```python
from build123d import *

# Parameters (mm, degrees)
SKETCH1_W               = 96.0628
SKETCH1_H               = 90.3478
PCB_DEPTH               = 1.6256
SKETCH5_R               = 1.5875
PCB_HOLES_DEPTH         = 66.957101229
SKETCH2_W               = 7.9756
SKETCH2_H               = 60.2234
PCI_104_CONNECTOR_DEPTH = 9.2964
SKETCH6_W               = 63.5
SKETCH6_H               = 7.366
PCB_EDGE_CONNS_DEPTH    = 5.461


with BuildPart() as part:
    # Sketch1 → PCB (new body)
    with BuildSketch(Plane.XY):
        Rectangle(SKETCH1_W, SKETCH1_H)
    extrude(amount=PCB_DEPTH)

    # Sketch5 → PCB_Holes (cut, through all)
    with BuildSketch(Plane.XY.offset(1.6256)):
        with Locations((-42.7736, 36.83)):
            Circle(SKETCH5_R)
        with Locations((42.9514, 40.005)):
            Circle(SKETCH5_R)
        with Locations((42.9514, -40.005)):
            Circle(SKETCH5_R)
        with Locations((-42.7736, -36.83)):
            Circle(SKETCH5_R)
    extrude(amount=-PCB_HOLES_DEPTH, mode=Mode.SUBTRACT)

    # Sketch2 → PCI-104_Connector (add)
    with BuildSketch(Plane.XY.offset(1.6256)):
        with Locations((-39.6494, 0.4064)):
            Rectangle(SKETCH2_W, SKETCH2_H)
    extrude(amount=PCI_104_CONNECTOR_DEPTH)

    # Sketch6 → PCB_Edge_Conns (add)
    with BuildSketch(Plane.XY.offset(1.6256)):
        with Locations((-3.5814, -46.0629)):
            Rectangle(SKETCH6_W, SKETCH6_H)
    extrude(amount=PCB_EDGE_CONNS_DEPTH)


solid = part.part
```
Source: CAD feature listing. Evaluate the final solid. Frame: model axes, mm. A direction names the side the tool comes from. Round coordinates to 2 decimals unless told otherwise and drop trailing zeros. Write each loop counter-clockwise with the first axis right and the second up, starting at its lowest first coordinate (ties: lowest second). Pieces come first, ordered by that corner, then holes. Notation, with made-up numbers: M 42.25,53.25 L 74.25,53.25 A19 cw 74.25,69.25 Z; hole C 62,-40 d8. An arc over 180 degrees is marked long. Use CSV: the item, a comma, the result in double quotes. Start each with the question number.
Q1. Cut plane B-B on z = 5.25. Output: boundary loops of the cut face in (x, y), plus the area to 3 significant figures.
Q2. Cut plane A-A on y = -36.83. Output: boundary loops of the cut face in (x, z), plus the area to 3 significant figures.
Q3. First-contact query: P1, Ø5, axis at x = 42.95, y = -40.01, coming from the +Z side; P2, Ø1.6, axis at x = 0, z = 5, coming from the +Y side; P3, Ø2.5, axis at x = -39.5, z = 8, coming from the +Y side; P4, Ø3, axis at x = 42.95, y = 40.01, coming from the +Z side. Flat tips, straight axial feed; report the tip coordinate or a pass-through.
Q4. Pull-direction query (Y, two-part tool) for faces 5 (the face through (-40, 1, 10.922)), 6 (the face through (43.684, 38.597, 0.824)), 7 (the face through (-4, -42.38, 4)); classes: +Y half, -Y half, draft (parallel to the pull), parting line (faces both ways), or undercut.
Q5. Line query: line 1 (Y direction, x = -30, z = 5.5); line 2 (X direction, y = -12.5, z = 2.75); line 3 (Z direction, x = 23.5, y = 27). Output: solid intervals per line, ascending. Write a range as from..to.
Q6. Cut plane C-C on x = -27.5. Output: boundary loops of the cut face in (y, z), plus the area to 3 significant figures.
Q7. Access query for faces 1 (the face through (-40, 30.518, 6)), 2 (the face through (-43.637, 0, 6)), 3 (the face through (-40, -29.705, 6)), 4 (the face through (28.169, -46, 4)). Directions: +Z, -Z, +X, -X, +Y, -Y. A direction counts if a zero-diameter tool reaches every point of the face in a straight line with its end or side. Return the directions, or none.
Q8. Cut plane D-D on y = 5.5. Output: boundary loops of the cut face in (x, z), plus the area to 3 significant figures.
Results found:
1,outline,"M -43.64,-29.71 L -35.66,-29.71 L -35.66,30.52 L -43.64,30.52 Z; M -35.33,-49.75 L 28.17,-49.75 L 28.17,-42.38 L -35.33,-42.38 Z"
1,area,"948 mm^2"
2,outline,"M -48.03,0 L -44.36,0 L -44.36,1.63 L -48.03,1.63 Z; M -41.19,0 L 48.03,0 L 48.03,1.63 L -41.19,1.63 Z"
2,area,"151 mm^2"
3,P1,"z = 1.63"
3,P2,"y = -42.38"
3,P3,"y = 30.52"
3,P4,"through"
4,face 5,"draft"
4,face 6,"undercut"
4,face 7,"+Y half"
5,line 1,"-49.75..-42.38"
5,line 2,"-43.64..-35.66"
5,line 3,"0..1.63"
6,outline,"M -49.75,1.63 L -45.17,1.63 L -45.17,0 L 45.17,0 L 45.17,1.63 L -42.38,1.63 L -42.38,7.09 L -49.75,7.09 Z"
6,area,"187 mm^2"
7,face 1,"+Z, +X, -X, +Y"
7,face 2,"+Z, -X, +Y, -Y"
7,face 3,"+Z, +X, -X, -Y"
7,face 4,"+Z, +X, +Y, -Y"
8,outline,"M -48.03,0 L 48.03,0 L 48.03,1.63 L -35.66,1.63 L -35.66,10.92 L -43.64,10.92 L -43.64,1.63 L -48.03,1.63 Z"
8,area,"230 mm^2"
